For this review, take the finished solid that the model builds, in its own axes (mm). Coordinates: 2 decimals unless noted, no trailing zeros. Write each loop counter-clockwise with the first axis right and the second up, starting at its lowest first coordinate (ties: lowest second). Pieces come first, ordered by that corner, then holes.
1) We need section C-C on y = 5. Write out the cut boundary in (x, z) (3 decimals), then the cut area to 3 significant figures.
2) We need section A-A on z = 120. Write out the cut boundary in (x, y).
3) We need section D-D on z = 68. Write out the cut boundary in (x, y), then the cut area to 3 significant figures.
4) To check wall thickness, follow line 1 along Y through (x, z) = (-53.25, 120); line 2 along Z through (x, y) = (-48.5, 3.25); line 3 along X through (y, z) = (8.5, 30). State the ranges of each line that lie inside material, in increasing order.
5) Insertion check: P1, Ø12, axis at x = -90.5, z = 86, coming from the -Y side; P2, Ø6, axis at x = -178.5, y = 5, coming from the +Z side; P3, Ø6, axis at y = 1.5, z = 70.5, coming from the +X side; P4, Ø1.5, axis at y = 1.5, z = 78, coming from the -X side. Each pin has a flat end and moves straight along its axis. Give the tip position at first contact, or say it passes through.
6) We need section B-B on x = -230. Write out the cut boundary in (y, z), then the cut area to 3 significant figures.
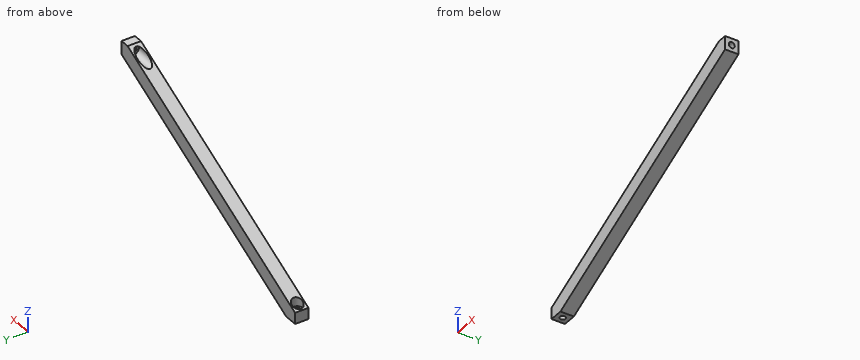
from build123d import *

# Parameters (mm, degrees)
BOSS_EXTRU_1_DEPTH      = 10
ESQUISSE4_R             = 2.1
ENL_V_MAT_EXTRU_1_DEPTH = 104
D_GAGEMENT_M41_D        = 4.5
ESQUISSE7_R             = 4
ENL_V_MAT_EXTRU_2_DEPTH = 12
ESQUISSE8_R             = 4
ENL_V_MAT_EXTRU_3_DEPTH = 28


with BuildPart() as part:
    # Esquisse1 → Boss.-Extru.1 (new body)
    with BuildSketch(Plane(origin=(0, 0, 0), x_dir=(1, 0, 0), z_dir=(0, 1, 0))):
        Polygon((-235, -22), (-235, -30.403916389), (-46.824994968, -125), (-40, -125), (-40, -115), (-225, -22), align=None)
    extrude(amount=BOSS_EXTRU_1_DEPTH)

    # Esquisse4 → Enlèv. mat.-Extru.1 (cut, through all)
    with BuildSketch(Plane(origin=(0, 0, 22), x_dir=(-1, 0, 0), z_dir=(0, 0, -1))):
        with Locations((230, 5)):
            Circle(ESQUISSE4_R)
    extrude(amount=-ENL_V_MAT_EXTRU_1_DEPTH, mode=Mode.SUBTRACT)

    # Dégagement M41 (through all)
    with Locations(Plane(origin=(-40, 0, 0), x_dir=(0, 0, -1), z_dir=(1, 0, 0))):
        with Locations((-120, 5)):
            Hole(D_GAGEMENT_M41_D / 2)

    # Esquisse7 → Enlèv. mat.-Extru.2 (cut)
    with BuildSketch(Plane(origin=(0, 0, 28), x_dir=(-1, 0, 0), z_dir=(0, 0, -1))):
        with Locations((230, 5)):
            Circle(ESQUISSE7_R)
    extrude(amount=-ENL_V_MAT_EXTRU_2_DEPTH, mode=Mode.SUBTRACT)

    # Esquisse8 → Enlèv. mat.-Extru.3 (cut)
    with BuildSketch(Plane(origin=(-46, 0, 0), x_dir=(0, 0, -1), z_dir=(1, 0, 0))):
        with Locations((-120, 5)):
            Circle(ESQUISSE8_R)
    extrude(amount=-ENL_V_MAT_EXTRU_3_DEPTH, mode=Mode.SUBTRACT)


solid = part.part
Result:
1. outline: (-235, 22) - (-232.1, 22) - (-232.1, 28) - (-234, 28) - (-234, 30.907) - (-235, 30.404) - close; (-227.9, 22) - (-225, 22) - (-40, 115) - (-40, 117.75) - (-46, 117.75) - (-46, 116) - (-64.728, 116) - (-226, 34.928) - (-226, 28) - (-227.9, 28) - close; (-48.814, 124) - (-46, 124) - (-46, 122.25) - (-40, 122.25) - (-40, 125) - (-46.825, 125) - close
1. area: 2,400 mm2
2. outline: (-56.77, 0) - (-40, 0) - (-40, 2.75) - (-46, 2.75) - (-46, 1) - (-56.77, 1) - close; (-56.77, 9) - (-46, 9) - (-46, 7.25) - (-40, 7.25) - (-40, 10) - (-56.77, 10) - close
3. outline: (-160.21, 0) - (-133.49, 0) - (-133.49, 10) - (-160.21, 10) - close
3. area: 267 mm2
4. line 1: y = 0 to 1, 9 to 10
4. line 2: z = 110.73 to 116.4, 123.6 to 124.16
4. line 3: x = -235 to -231.94, -228.06 to -209.09
5. P1: stops at y = 0
5. P2: stops at z = 60.31
5. P3: stops at x = -122.55
5. P4: stops at x = -141.81
6. outline: (0, 22) - (2.9, 22) - (2.9, 28) - (1, 28) - (1, 32.92) - (0, 32.92) - close; (7.1, 22) - (10, 22) - (10, 32.92) - (9, 32.92) - (9, 28) - (7.1, 28) - close
6. area: 44.6 mm2
